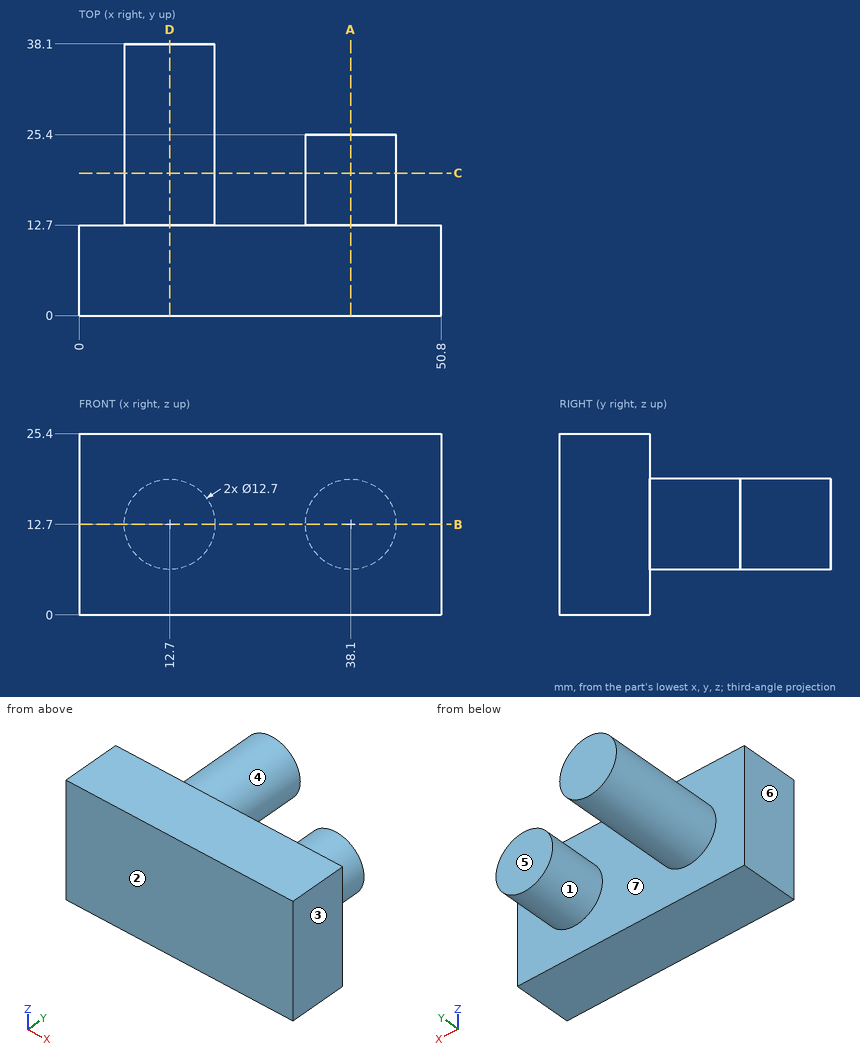
For this review, use the dimensioned drawing (mm, ordinates from the lowest corner) and the shaded views. A direction names the side the tool comes from. Round coordinates to 2 decimals unless told otherwise and drop trailing zeros. Write each loop counter-clockwise with the first axis right and the second up, starting at its lowest first coordinate (ties: lowest second). Pieces come first, ordered by that corner, then holes. Notation, with made-up numbers: (70, 18) - (126, 18) arc R25 ccw to (126, 49) - close; hole circle Ø10 at (33, 41). An arc over 180 degrees is marked (long way). Use a Markdown table: item, result.
Q1. We need section D-D (x = 12.7). Give the boundary of the cut face in (y, z).
Derived:
| item | result |
|---|---|
| outline | (0, 0) - (12.7, 0) - (12.7, 6.35) - (38.1, 6.35) - (38.1, 19.05) - (12.7, 19.05) - (12.7, 25.4) - (0, 25.4) - close |
Q2. The part is to be moulded in two halves that separate along X. For the marked faces 1, 2, 3 and 4, say which applies: pulls with the +X half, pulls with the -X half, needs draft (parallel to the pull), parting line crosses it, or undercut.
Derived:
| item | result |
|---|---|
| face 1 | undercut |
| face 2 | needs draft |
| face 3 | pulls with the +X half |
| face 4 | undercut |
Q3. We need section A-A (x = 38.1). Give the boundary of the cut face in (y, z).
Derived:
| item | result |
|---|---|
| outline | (0, 0) - (12.7, 0) - (12.7, 6.35) - (25.4, 6.35) - (25.4, 19.05) - (12.7, 19.05) - (12.7, 25.4) - (0, 25.4) - close |
Q4. Wall thickness on line 1 along X through (y, z) = (33.5, 13); line 2 along Y through (x, z) = (47, 23.5); line 3 along Y through (x, z) = (40, 11.75): over which ranges is each line inside the solid? List them lowest first.
Derived:
| item | result |
|---|---|
| line 1 | x = 6.36 to 19.04 |
| line 2 | y = 0 to 12.7 |
| line 3 | y = 0 to 25.4 |
Q5. We need section C-C (y = 20). Give the boundary of the cut face in (x, z), plus the area to 3 significant figures.
Derived:
| item | result |
|---|---|
| outline | circle Ø12.7 at (12.7, 12.7); circle Ø12.7 at (38.1, 12.7) |
| area | 253 mm2 |
Q6. Clearance check with flat-ended pins moving along their axes: pin 1 (1 mm diameter, centred on x = 36, z = 22.5, fed in from -Y); pin 2 (12 mm diameter, centred on y = 31, z = 20, fed in from -X); pin 3 (6 mm diameter, centred on y = 30, z = 22.5, fed in from +X); pin 4 (1.5 mm diameter, centred on x = 6.5, y = 34, fed in from -Z). State where each tip first meets the part, or that it passes through.
Derived:
| item | result |
|---|---|
| pin 1 | stops at y = 0 |
| pin 2 | stops at x = 6.48 |
| pin 3 | passes through |
| pin 4 | stops at z = 9.44 |
Q7. We need section B-B (z = 12.7). Give the boundary of the cut face in (x, y), plus the area to 3 significant figures.
Derived:
| item | result |
|---|---|
| outline | (0, 0) - (50.8, 0) - (50.8, 12.7) - (44.45, 12.7) - (44.45, 25.4) - (31.75, 25.4) - (31.75, 12.7) - (19.05, 12.7) - (19.05, 38.1) - (6.35, 38.1) - (6.35, 12.7) - (0, 12.7) - close |
| area | 1,130 mm2 |
Q8. Machinability: for the marked faces 5, 6 and 7, which of the approach directions +Z, -Z, +X, -X, +Y, -Y give a long, thin tool a straight path to every point of the face, cutting with its end or side? Answer none if there is none.
Derived:
| item | result |
|---|---|
| face 5 | +Z, -Z, +X, +Y |
| face 6 | +Z, -Z, -X, +Y, -Y |
| face 7 | +Y |
